For this review, use the dimensioned drawing (mm, ordinates from the lowest corner) and the shaded views. Coordinates: 2 decimals unless noted, no trailing zeros. Write each loop counter-clockwise with the first axis right and the second up, starting at its lowest first coordinate (ties: lowest second). Pieces come first, ordered by that corner, then holes.
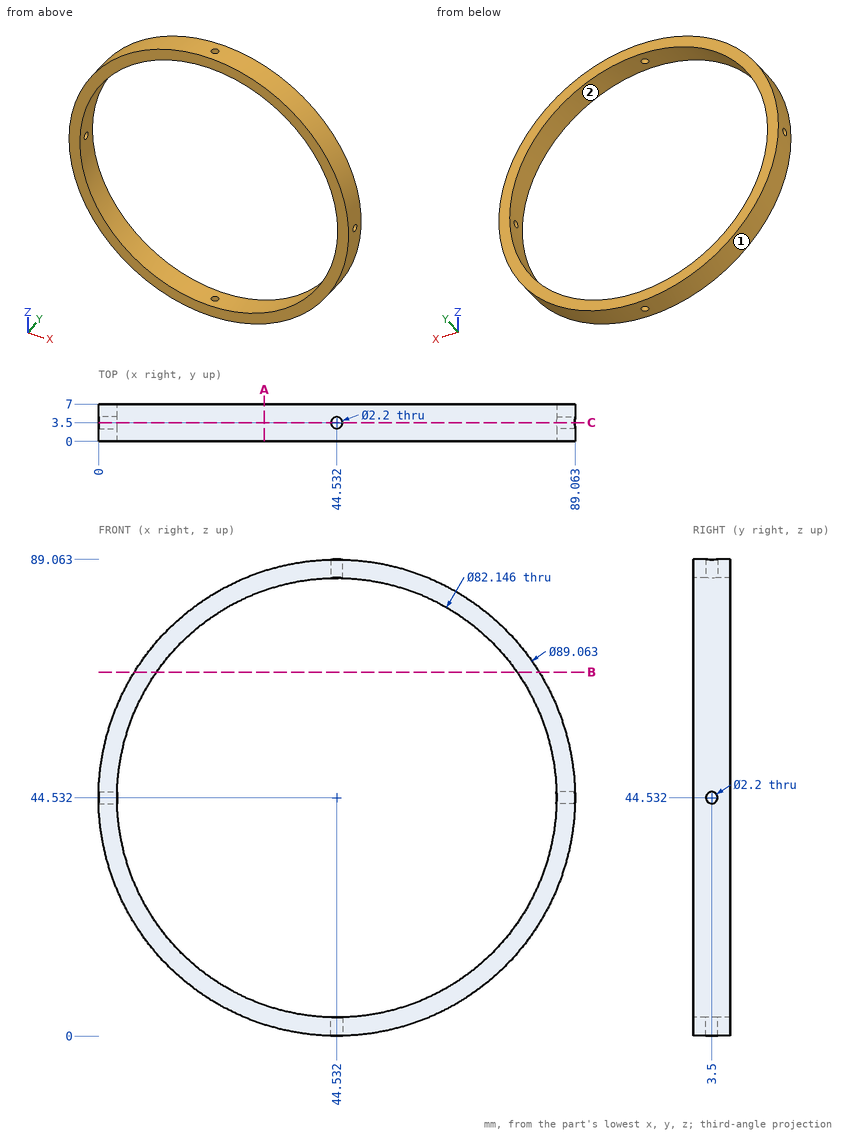
(1) Consider section C-C (y = 3.5). State how many separate pieces and enclosed holes the cut face has.
(2) Mouldability with a two-part tool opening along Z and no side actions: class the marked faces 1 and 2 as +Z half, -Z half, draft (parallel to the pull), parting line (faces both ways), or undercut.
(3) Wall thickness on line 1 (Z direction, x = 77, y = 3.5) (1 decimal); line 2 (X direction, y = 1.5, z = 63.5); line 3 (X direction, y = 5.25, z = 51): over which ranges is each line inside the solid? List them lowest first.
(4) Consider section B-B (z = 68). Give the boundary of the cut face in (x, y) (1 decimal).
(5) Consider section A-A (x = 31). Give the boundary of the cut face in (y, z) (1 decimal).
(6) Insertion check: pin 1 Ø2 at (x, y) = (50, 6) entering from +Z; pin 2 Ø3 at (y, z) = (2, 27) entering from -X (1 decimal); pin 3 Ø1 at (x, y) = (31.5, 3) entering from +Z. Each pin has a flat end and moves straight along its axis. Give the tip position at first contact, or say it passes through.
Results:
1. separate pieces: 4
1. enclosed holes: 0
2. face 1: parting line
2. face 2: undercut
3. line 1: z = 14.1 to 19.4, 69.7 to 75
3. line 2: x = 4.24 to 8.1, 80.96 to 84.82
3. line 3: x = 0.47 to 3.97, 85.09 to 88.59
4. outline: (6.7, 0) - (10.8, 0) - (10.8, 7) - (6.7, 7) - close; (78.2, 0) - (82.4, 0) - (82.4, 7) - (78.2, 7) - close
5. outline: (0, 2.1) - (7, 2.1) - (7, 5.8) - (0, 5.8) - close; (0, 83.3) - (7, 83.3) - (7, 87) - (0, 87) - close
6. pin 1: stops at z = 88.84
6. pin 2: stops at x = 3
6. pin 3: stops at z = 87.26
